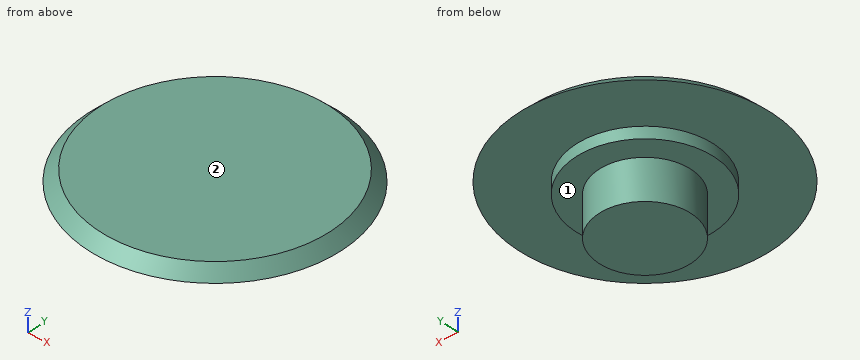
from build123d import *

# Parameters (mm, degrees)
F0_R     = 4
F1_DEPTH = 3.5
F2_R     = 6
F3_DEPTH = 1
F4_R     = 11
F5_DEPTH = 1
F7_SIZE  = 0.99999


# Not quite as in the source:
# - a fillet or chamfer is up to 0.001 mm smaller than in the source, because OpenCascade refuses the exact size


with BuildPart() as f1:
    # F0 (on Top) → F1 (new body)
    with BuildSketch(Plane.XY):
        Circle(F0_R)
    extrude(amount=F1_DEPTH)

    # F2 (on face) → F3 (join)
    with BuildSketch(Plane.XY.offset(3.5)):
        Circle(F2_R)
    extrude(amount=F3_DEPTH)

    # F4 (on face) → F5 (join)
    with BuildSketch(Plane.XY.offset(4.5)):
        Circle(F4_R)
    extrude(amount=F5_DEPTH)

    # F7 (size 1 in the source; OpenCascade refuses exactly that, so slightly less here)
    f7_edges = [f1.edges().sort_by_distance(p)[0] for p in [
        (-11, 0, 5.5),
    ]]
    chamfer(f7_edges, length=F7_SIZE)


solid = f1.part
Can you work these out from the model? Positions are in its coordinate system, mm. Face numbers are marked on the shaded views. A direction names the side the tool comes from. Round coordinates to 2 decimals unless told otherwise and drop trailing zeros. Loops run counter-clockwise (first coordinate to the right, second up) from the corner with the lowest first, then second, coordinate; pieces in that order, holes last. Notation, with made-up numbers: (80, -20.5) - (88, -20.5) arc R24 ccw to (88, -9.5) - close; hole circle Ø2 at (11.5, 81). An arc over 180 degrees is marked (long way). Answer in a Markdown table with one row per item. Add a question column.
Q1. I want a section at C-C on z = 2.15. List the corners of the cut face in (x, y) for me, and give its area (3 significant figures).
Q2. I need wall thicknesses on L1, parallel to Z at x = 2.5, y = 3.75; L2, parallel to Z at x = -1, y = 6.75; L3, parallel to Y at x = 0.25, z = 1.65. Which ranges of each line are inside material? Lowest first, please.
Q3. Which directions (+Z, -Z, +X, -X, +Y, -Y) give clear straight access to the entire face, cutting with the end or side of a thin tool? Please do the marked faces 1 and 2.
Q4. I want a section at D-D on z = 4.9. List the corners of the cut face in (x, y) for me.
Q5. For pin 1 Ø2 at (x, y) = (5.5, 2.5) entering from -Z, with a flat end and sliding along its axis, tell me the tip position at first contact or that it passes through.
A:
| question | item | result |
|---|---|---|
| 1 | outline | circle Ø8 at (0, 0) |
| 1 | area | 50.3 mm^2 |
| 2 | L1 | 3.5 to 5.5 |
| 2 | L2 | 4.5 to 5.5 |
| 2 | L3 | -3.99 to 3.99 |
| 3 | face 1 | -Z |
| 3 | face 2 | +Z, +X, -X, +Y, -Y |
| 4 | outline | circle Ø21.2 at (0, 0) |
| 5 | pin 1 | z = 3.5 |
